```python
from build123d import *
from build123d.topology import SkipClean

# Parameters (mm, degrees)
CROQUIS1_R              = 52.45
CROQUIS1_R_2            = 44.45
SALIENTE_EXTRUIR1_DEPTH = 227
CROQUIS2_R              = 52.45
CROQUIS2_R_2            = 44.45
SALIENTE_EXTRUIR2_DEPTH = 119
CROQUIS3_R              = 44.45
CORTAR_EXTRUIR1_DEPTH   = 227


with BuildPart() as part:
    # Croquis1 → Saliente-Extruir1 (new body)
    with BuildSketch(Plane(origin=(0, 0, 0), x_dir=(0, 0, -1), z_dir=(1, 0, 0))):
        with Locations(Location((0, 0, 0), (0, 0, 180))):
            Circle(CROQUIS1_R)
        with Locations(Location((0, 0, 0), (0, 0, 180))):
            Circle(CROQUIS1_R_2, mode=Mode.SUBTRACT)
    extrude(amount=SALIENTE_EXTRUIR1_DEPTH)

    # Croquis2 → Saliente-Extruir2 (add)
    with BuildSketch(Plane(origin=(0, 0, 0), x_dir=(1, 0, 0), z_dir=(0, 1, 0))):
        with Locations(Location((113.5, 0, 0), (0, 0, 270))):
            Circle(CROQUIS2_R)
        with Locations(Location((113.5, 0, 0), (0, 0, 90))):
            Circle(CROQUIS2_R_2, mode=Mode.SUBTRACT)
    extrude(amount=SALIENTE_EXTRUIR2_DEPTH)

    # Croquis3 → Cortar-Extruir1 (cut)
    with SkipClean():  # the faces are left unmerged after this step: merging them gives an invalid solid
        with BuildSketch(Plane.ZY):
            Circle(CROQUIS3_R)
        extrude(amount=-CORTAR_EXTRUIR1_DEPTH, mode=Mode.SUBTRACT)


solid = part.part
```
For this review, take the finished solid that the model builds, in its own axes (mm). A direction names the side the tool comes from. Give positions to 0.01 mm unless a question says otherwise; leave off trailing zeros. Write each loop counter-clockwise with the first axis right and the second up, starting at its lowest first coordinate (ties: lowest second). Pieces come first, ordered by that corner, then holes. Notation, with made-up numbers: M -26,18.5 L 25,18.5 A18 cw 25,43.5 Z; hole C 48.25,-30 d3. An arc over 180 degrees is marked long. Answer as a JSON object with one key per item and string values. Group by question number.
Item 1: For pin 1 Ø10 at (x, y) = (85.5, -15) entering from -Z; pin 2 Ø4 at (x, z) = (45, -20) entering from +Y; pin 3 Ø10 at (x, y) = (60, 99.5) entering from -Z, all flat-tipped, find the tip position at first contact; note any pin that passes through.
Item 2: Draft analysis for pull direction Z (two halves, no side actions). For faces 3 (the cylindrical face through (83.5, 82.9, 32.8)), 4 (the flat face through (125.4, 119, -43)), 5 (the cylindrical face through (111.9, -30, -32.8)), 6 (the cylindrical face through (148.9, 71.9, -38.7)), state which applies: +Z half, -Z half, draft (parallel to the pull), parting line (faces both ways), or undercut.
Item 3: Consider section A-A on z = 0. Write out the cut boundary in (x, y).
Item 4: Tool access review of faces 1 (the cylindrical face through (111.911, -52.004, -6.828)), 2 (the flat face through (0, -12, -43)): name each direction out of +Z, -Z, +X, -X, +Y, -Y from which nothing blocks a thin tool from reaching the whole face with its end or side.
Item 5: Consider section D-D on x = 81. Write out the cut boundary in (y, z).
Item 6: Consider section C-C on y = 102. Write out the cut boundary in (x, z).
Item 7: Consider section B-B on x = 113.5. Write out the cut boundary in (y, z), plus the area to 3 significant figures.
Item 8: For probe 1 along Y at (x, z) = (109, 0); probe 2 along X at (y, z) = (88, 0); probe 3 along Y at (x, z) = (69, 0), list the stretches that pass through material, from the lowest coordinate up. Write a range as [from, to].
Check result:
{
 "1": {"pin 1": "stops at z = -51.49", "pin 2": "stops at y = 49.26", "pin 3": "stops at z = -19.97"},
 "2": {"face 3": "undercut", "face 4": "draft", "face 5": "undercut", "face 6": "parting line"},
 "3": {"outline": "M 0,-52.45 L 227,-52.45 L 227,-44.45 L 0,-44.45 Z; M 0,44.45 L 227,44.45 L 227,52.45 L 165.95,52.45 L 165.95,119 L 157.95,119 L 157.95,52.45 L 69.05,52.45 L 69.05,119 L 61.05,119 L 61.05,52.45 L 0,52.45 Z"},
 "4": {"face 1": "none", "face 2": "+Z, -Z, -X, +Y, -Y"},
 "5": {"outline": "M 32.5,-41.17 L 119,-41.17 L 119,-30.32 L 42.8,-30.32 A52.45 ccw 42.8,30.32 L 119,30.32 L 119,41.17 L 32.5,41.17 A52.45 ccw long Z; hole C 0,0 d88.9"},
 "6": {"outline": "C 113.5,0 d104.9; hole C 113.5,0 d88.9"},
 "7": {"outline": "M 0,-52.45 L 119,-52.45 L 119,-44.45 L 27.84,-44.45 A52.45 ccw 27.84,44.45 L 119,44.45 L 119,52.45 L 0,52.45 A52.45 ccw Z; hole C 0,0 d88.9", "area": "4,040 mm^2"},
 "8": {"probe 1": "y = [-52.45, -44.45], [44.45, 52.45]", "probe 2": "x = [61.05, 69.05], [157.95, 165.95]", "probe 3": "y = [-52.45, -44.45], [44.45, 119]"}
}
